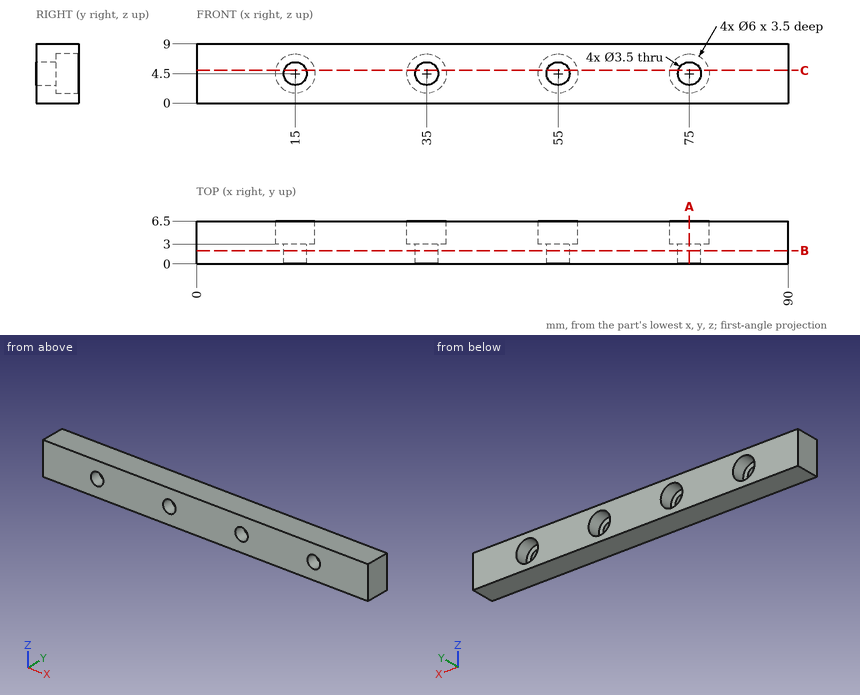
Job drawing, mm, ordinate dimensions from the low corner. One solid piece. Coordinates: 2 decimals unless noted, no trailing zeros. Loops run counter-clockwise (first coordinate to the right, second up) from the corner with the lowest first, then second, coordinate; pieces in that order, holes last. Notation, with made-up numbers: (71.25, 85) - (128.25, 85) arc R13 ccw to (128.25, 98) - close; hole circle Ø5 at (22.5, 48). An arc over 180 degrees is marked (long way). Answer as a JSON object with one key per item and string values. Group by question number.
(1) Cut at C-C (z = 5). State how many separate pieces and enclosed holes the cut face has, then the cut area to 3 significant figures.
(2) Probe line 1 along X through (y, z) = (1.6, 4.5); line 2 along X through (y, z) = (4.35, 4.5); line 3 along Y through (x, z) = (36.5, 6.5). List the from-to ranges inside material, lowest first.
(3) Flat gauge pin, fed straight in: pin 1 (3 mm diameter, centred on x = 15, z = 5, fed in from +Y). Where does the tip first touch, or does it go through?
(4) Cut at B-B (y = 2). Give the cut face in (x, z), then the cut area to 3 significant figures.
(5) Cut at A-A (x = 75). Give the cut face in (y, z), then the cut area to 3 significant figures.
Geometry says:
{
 "1": {"separate pieces": "5", "enclosed holes": "0", "area": "462 mm^2"},
 "2": {"line 1": "x = 0 to 13.25, 16.75 to 33.25, 36.75 to 53.25, 56.75 to 73.25, 76.75 to 90", "line 2": "x = 0 to 12, 18 to 32, 38 to 52, 58 to 72, 78 to 90", "line 3": "y = 0 to 3"},
 "3": {"pin 1": "stops at y = 3"},
 "4": {"outline": "(0, 0) - (90, 0) - (90, 9) - (0, 9) - close; hole circle Ø3.5 at (15, 4.5); hole circle Ø3.5 at (35, 4.5); hole circle Ø3.5 at (55, 4.5); hole circle Ø3.5 at (75, 4.5)", "area": "772 mm^2"},
 "5": {"outline": "(0, 0) - (6.5, 0) - (6.5, 1.5) - (3, 1.5) - (3, 2.75) - (0, 2.75) - close; (0, 6.25) - (3, 6.25) - (3, 7.5) - (6.5, 7.5) - (6.5, 9) - (0, 9) - close", "area": "27.0 mm^2"}
}
